Work out the finished part from the listing and answer in its coordinate system (mm). Face numbers are marked on the shaded views. Round coordinates to 2 decimals unless told otherwise and drop trailing zeros. Write each loop counter-clockwise with the first axis right and the second up, starting at its lowest first coordinate (ties: lowest second). Pieces come first, ordered by that corner, then holes. Notation, with made-up numbers: (-37, 33.25) -> (18, 33.25) arc R33 cw to (18, 66.25) -> close; hole circle Ø7 at (79, 65.25). An arc over 180 degrees is marked (long way). One line per item, written item: value.
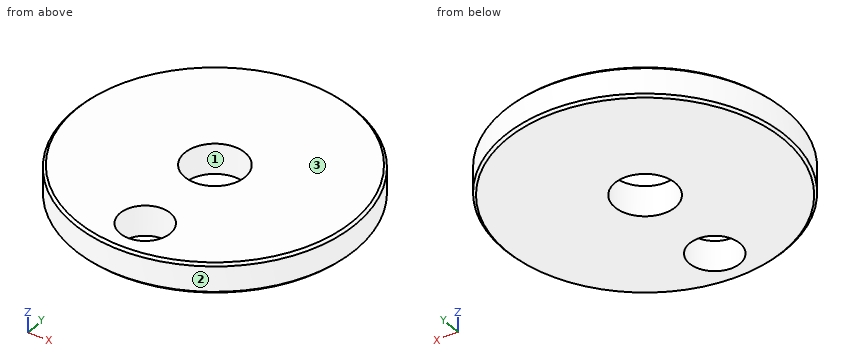
```python
from build123d import *

# Parameters (mm, degrees)
F0_R     = 22.225
F0_R_2   = 3.9751
F0_R_3   = 4.7625
F1_DEPTH = 4.7752
F2_SIZE  = 0.381


with BuildPart() as f1:
    # F0 (on Top) → F1 (new body)
    with BuildSketch(Plane.XY):
        Circle(F0_R)
        with Locations((0, -15.875)):
            Circle(F0_R_2, mode=Mode.SUBTRACT)
        Circle(F0_R_3, mode=Mode.SUBTRACT)
    extrude(amount=F1_DEPTH)

    # F2
    f2_edges = [f1.edges().sort_by_distance(p)[0] for p in [
        (-22.225, 0, 4.7752),
        (-22.225, 0, 0),
    ]]
    chamfer(f2_edges, length=F2_SIZE)


solid = f1.part
```
(1) For a pull along Y with two mould halves and no side action, classify the marked faces 1, 2 and 3 as pulls with the +Y half, pulls with the -Y half, needs draft (parallel to the pull), parting line crosses it, or undercut.
Reported:
face 1: undercut
face 2: parting line crosses it
face 3: needs draft
(2) Consider probe 1 along Y at (x, z) = (0, 1.25) (1 decimal); probe 2 along X at (y, z) = (0.5, 1.8); probe 3 along X at (y, z) = (-1.5, 4.1). Determine where each line is inside the solid, lowest interval first.
Reported:
probe 1: y = -22.2 to -19.9, -11.9 to -4.8, 4.8 to 22.2
probe 2: x = -22.22 to -4.74, 4.74 to 22.22
probe 3: x = -22.17 to -4.52, 4.52 to 22.17
(3) Find section C-C on z = 2.6. Give the number of separate pieces and of enclosed holes in the cut face, plus the area to 3 significant figures.
Reported:
separate pieces: 1
enclosed holes: 2
area: 1,430 mm2
(4) Find section B-B on y = 0. Give the vertices of the cut face in (x, z) (1 decimal).
Reported:
outline: (-22.2, 0.4) -> (-21.8, 0) -> (-4.8, 0) -> (-4.8, 4.8) -> (-21.8, 4.8) -> (-22.2, 4.4) -> close; (4.8, 0) -> (21.8, 0) -> (22.2, 0.4) -> (22.2, 4.4) -> (21.8, 4.8) -> (4.8, 4.8) -> close
(5) Find section A-A on x = 0. Give the vertices of the cut face in (y, z) (1 decimal), plus the area to 3 significant figures.
Reported:
outline: (-22.2, 0.4) -> (-21.8, 0) -> (-19.9, 0) -> (-19.9, 4.8) -> (-21.8, 4.8) -> (-22.2, 4.4) -> close; (-11.9, 0) -> (-4.8, 0) -> (-4.8, 4.8) -> (-11.9, 4.8) -> close; (4.8, 0) -> (21.8, 0) -> (22.2, 0.4) -> (22.2, 4.4) -> (21.8, 4.8) -> (4.8, 4.8) -> close
area: 129 mm2
